Can you work these out from the model? Positions are in its coordinate system, mm. A direction names the side the tool comes from. Round coordinates to 2 decimals unless told otherwise and drop trailing zeros. Write each loop counter-clockwise with the first axis right and the second up, starting at its lowest first coordinate (ties: lowest second). Pieces come first, ordered by that corner, then holes.
Q1. I'm going to push a flat-ended pin straight in: pin 1 Ø0.9 at (y, z) = (36, 1.5) entering from +X. Where does the tip first touch, or does it pass through?
Q2. If we section it at B-B (z = -1): Please give me the cut outline in (x, y).
Q3. If we section it at A-A (y = 37): Please give me the cut outline in (x, z), plus the area to 4 significant figures.
Q4. Please list where these lines run through material, in increasing order: line 1 along X through (y, z) = (37.5, -0.1); line 2 along Y through (x, z) = (35, 1.5).
Q5. For faces 1 (the flat face through (49, 35, 0)), 2 (the flat face through (50.75, 35, 1)), 3 (the flat face through (35, 19.25, 1)), which set-ups out of +Z, -Z, +X, -X, +Y, -Y let a thin tool reach every point of the face, with its end or its side?
Q6. If we section it at D-D (x = 53): Please give me the cut outline in (y, z), plus the area to 3 significant figures.
Q7. We'd pull the mould along X, two halves only. Please class faces 4 (the flat face through (35, 21, 0)), 5 (the flat face through (35, 50.75, 1)), 6 (the cylindrical face through (0.713, 69.248, -1.521)): +X half, -X half, draft (parallel to the pull), parting line (faces both ways), or undercut.
from build123d import *

# Parameters (mm, degrees)
SKETCH001_W  = 70
SKETCH001_H  = 70
PAD001_DEPTH = 3
FILLET001_R  = 2.5
SKETCH002_W  = 31.5
SKETCH002_H  = 31.5
PAD002_DEPTH = 3
SKETCH003_W  = 28
SKETCH003_H  = 28
POCKET_DEPTH = 6.001


with BuildPart() as part:
    # Sketch001 → Pad001 (new body)
    with BuildSketch(Plane.XY):
        with Locations((35, 35)):
            Rectangle(SKETCH001_W, SKETCH001_H)
    extrude(amount=-PAD001_DEPTH)

    # Fillet001
    fillet001_edges = [part.edges().sort_by_distance(p)[0] for p in [
        (70, 70, -1.5),
        (0, 70, -1.5),
        (70, 0, -1.5),
        (0, 0, -1.5),
    ]]
    fillet(fillet001_edges, radius=FILLET001_R)

    # Sketch002 (on Face2 of Fillet001) → Pad002 (join)
    with BuildSketch(Plane.XY):
        with Locations((35, 35)):
            Rectangle(SKETCH002_W, SKETCH002_H)
    extrude(amount=PAD002_DEPTH)

    # Sketch003 (on Face15 of Pad002) → Pocket (cut, through all)
    with BuildSketch(Plane.XY.offset(3)):
        with Locations((35, 35)):
            Rectangle(SKETCH003_W, SKETCH003_H)
    extrude(amount=-POCKET_DEPTH, mode=Mode.SUBTRACT)


solid = part.part
A:
1. pin 1: stops at x = 50.75
2. outline: (0, 2.5) arc R2.5 ccw to (2.5, 0) - (67.5, 0) arc R2.5 ccw to (70, 2.5) - (70, 67.5) arc R2.5 ccw to (67.5, 70) - (2.5, 70) arc R2.5 ccw to (0, 67.5) - close; hole (21, 21) - (49, 21) - (49, 49) - (21, 49) - close
3. outline: (0, -3) - (21, -3) - (21, 3) - (19.25, 3) - (19.25, 0) - (0, 0) - close; (49, -3) - (70, -3) - (70, 0) - (50.75, 0) - (50.75, 3) - (49, 3) - close
3. area: 136.5 mm2
4. line 1: x = 0 to 21, 49 to 70
4. line 2: y = 19.25 to 21, 49 to 50.75
5. face 1: +Z, -Z
5. face 2: +Z, +X, +Y, -Y
5. face 3: +Z, +X, -X, -Y
6. outline: (0, -3) - (70, -3) - (70, 0) - (0, 0) - close
6. area: 210 mm2
7. face 4: undercut
7. face 5: draft
7. face 6: -X half
